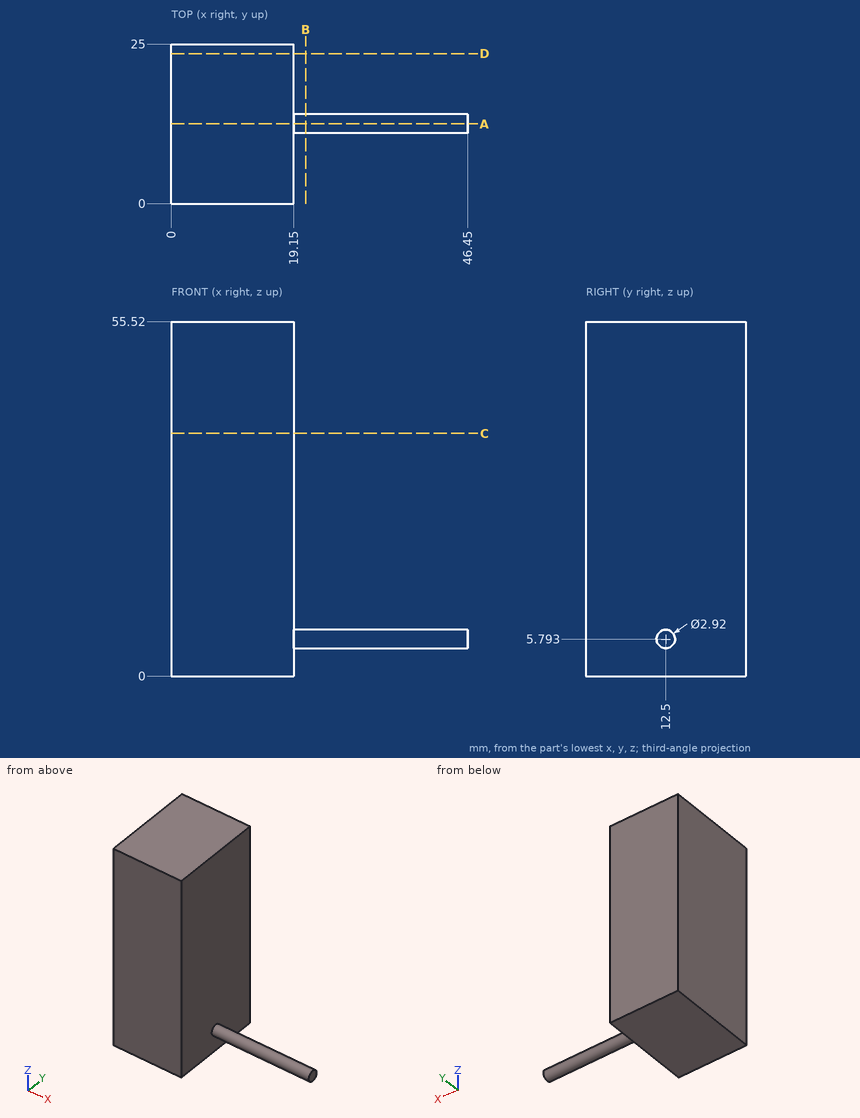
Here's the drawing with two shaded views (mm, measured from the low corner). I have some questions. Round coordinates to 2 decimals unless told otherwise and drop trailing zeros. Loops run counter-clockwise (first coordinate to the right, second up) from the corner with the lowest first, then second, coordinate; pieces in that order, holes last. Notation, with made-up numbers: (-21.75, -35.75) - (19.25, -35.75) arc R34 ccw to (19.25, -1.75) - close; hole circle Ø11 at (78, 77). An arc over 180 degrees is marked (long way). Write item = value, one per line.
1) Imagine slicing it at A-A (y = 12.5). Please give me the cut outline in (x, z), and give its area (3 significant figures).
Computed:
outline = (0, 0) - (19.15, 0) - (19.15, 4.33) - (46.45, 4.33) - (46.45, 7.25) - (19.15, 7.25) - (19.15, 55.52) - (0, 55.52) - close
area = 1,140 mm2
2) Imagine slicing it at B-B (x = 21). Please give me the cut outline in (y, z).
Computed:
outline = circle Ø2.92 at (12.5, 5.79)
3) I'm going to push flat-ended pins straight in: P1, Ø7.5, axis at y = 18, z = 21.5, coming from the +X side; P2, Ø5, axis at x = 23, z = 39, coming from the -Y side; P3, Ø6, axis at x = 36.5, y = 15.5, coming from the +Z side. Where does each tip first touch, or does it pass through?
Computed:
P1 = 19.15
P2 = through
P3 = 7.25
4) I need wall thicknesses on line 1 along X through (y, z) = (5, 14); line 2 along Z through (x, y) = (27.5, 12.5). Which ranges of each line are inside material? Lowest first, please. Write a range as from..to.
Computed:
line_1 = 0..19.15
line_2 = 4.33..7.25
5) Imagine slicing it at D-D (y = 23.5). Please give me the cut outline in (x, z).
Computed:
outline = (0, 0) - (19.15, 0) - (19.15, 55.52) - (0, 55.52) - close
6) Imagine slicing it at C-C (z = 38). Please give me the cut outline in (x, y), and give its area (3 significant figures).
Computed:
outline = (0, 0) - (19.15, 0) - (19.15, 25) - (0, 25) - close
area = 479 mm2
